from build123d import *

# Parameters (mm, degrees)
F1_DEPTH       = 18
F2_D           = 10
F3_D           = 10
F5_D           = 4
F5_CSINK_D     = 8.2
F5_CSINK_ANGLE = 90
F7_D           = 3
F7_DEPTH       = 20
F7_TIP         = 0.9012909285
F9_D           = 3
F9_DEPTH       = 20
F9_TIP         = 0.9012909285
F11_D          = 3
F11_DEPTH      = 20
F11_TIP        = 0.9012909285


with BuildPart() as f1:
    # F0 (on Right) → F1 (new body)
    with BuildSketch(Plane.YZ):
        Polygon((0, 230), (0, 0), (135, 0), (135, 206.1958576044), align=None)
    extrude(amount=F1_DEPTH)

    # F2 (through all)
    with Locations(Plane(origin=(0, 0, 0), x_dir=(0, 1, 0), z_dir=(-1, 0, 0))):
        with Locations((37.5, -170), (67.5, -170), (97.5, -170)):
            Hole(F2_D / 2)

    # F3 (through all)
    with Locations(Plane(origin=(0, 0, 0), x_dir=(0, 1, 0), z_dir=(-1, 0, 0))):
        with Locations((52.5, -190), (82.5, -190)):
            Hole(F3_D / 2)

    # F5 (through all)
    with Locations(Plane.YZ.offset(18)):
        with Locations((25, 27)):
            CounterSinkHole(F5_D / 2, F5_CSINK_D / 2, counter_sink_angle=F5_CSINK_ANGLE)

    # F7
    with Locations(Plane(origin=(0, 135, 0), x_dir=(-1, 0, 0), z_dir=(0, 1, 0))):
        with Locations((-9, 27), (-9, 106), (-9, 185)):
            Hole(F7_D / 2, depth=F7_DEPTH)
            with Locations((0, 0, -(F7_DEPTH + F7_TIP / 2))):  # 118° drill point
                Cone(0, F7_D / 2, F7_TIP, mode=Mode.SUBTRACT)

    # F9
    with Locations(Plane.XZ):
        with Locations((9, 197), (9, 112), (9, 27)):
            Hole(F9_D / 2, depth=F9_DEPTH)
            with Locations((0, 0, -(F9_DEPTH + F9_TIP / 2))):  # 118° drill point
                Cone(0, F9_D / 2, F9_TIP, mode=Mode.SUBTRACT)

    # F11
    with Locations(Plane(origin=(0, 39.3323164825, 223.0646513904), x_dir=(1, 0, 0), z_dir=(0, 0.1736481777, 0.984807753))):
        with Locations((9, -10.8564882588), (9, 79.1435117412)):
            Hole(F11_D / 2, depth=F11_DEPTH)
            with Locations((0, 0, -(F11_DEPTH + F11_TIP / 2))):  # 118° drill point
                Cone(0, F11_D / 2, F11_TIP, mode=Mode.SUBTRACT)


solid = f1.part
The model under review builds one solid part; all positions refer to its coordinate system, in mm. Coordinates: 2 decimals unless noted, no trailing zeros. Write each loop counter-clockwise with the first axis right and the second up, starting at its lowest first coordinate (ties: lowest second). Pieces come first, ordered by that corner, then holes. Notation, with made-up numbers: (62, -15) - (76, -15) arc R9 cw to (76, -10) - close; hole circle Ø8 at (-19, -28). An arc over 180 degrees is marked (long way). Answer as a JSON object with one key per item and string values. Group by question number.
1. Add section B-B (y = 37.5). Give the boundary of the cut face in (x, z).
2. Clearance check with flat-ended pins moving along their axes: pin 1 Ø2.5 at (y, z) = (25, 27) entering from -X; pin 2 Ø2.5 at (x, z) = (9, 27) entering from +Y; pin 3 Ø4 at (x, y) = (8.5, 41) entering from +Z; pin 4 Ø1.8 at (x, z) = (9, 112) entering from -Y. State where each tip first meets the part, or that it passes through.
3. Mouldability with a two-part tool opening along Z and no side actions: class faces 1 (the face through (9.126, 68.151, 165.043)), 2 (the face through (0, 67, 117)), 3 (the face through (9, 67, 0)) as pulls with the +Z half, pulls with the -Z half, needs draft (parallel to the pull), parting line crosses it, or undercut.
4. Add section A-A (z = 170). Give the boundary of the cut face in (x, y).
5. To check wall thickness, follow probe 1 along Y at (x, z) = (13.75, 190); probe 2 along Y at (x, z) = (5.25, 170); probe 3 along X at (y, z) = (14.75, 112). State the ranges of each line that lie inside material, in increasing order.
6. Add section C-C (y = 123.5). Give the boundary of the cut face in (x, z).
7. Add section D-D (y = 82). Give the boundary of the cut face in (x, z).
Findings:
{
 "1": {"outline": "(0, 0) - (18, 0) - (18, 165) - (0, 165) - close; (0, 175) - (18, 175) - (18, 223.39) - (0, 223.39) - close"},
 "2": {"pin 1": "through", "pin 2": "y = 114.85", "pin 3": "z = 223.12", "pin 4": "y = 20.36"},
 "3": {"face 1": "undercut", "face 2": "needs draft", "face 3": "pulls with the -Z half"},
 "4": {"outline": "(0, 0) - (18, 0) - (18, 32.5) - (0, 32.5) - close; (0, 42.5) - (18, 42.5) - (18, 62.5) - (0, 62.5) - close; (0, 72.5) - (18, 72.5) - (18, 92.5) - (0, 92.5) - close; (0, 102.5) - (18, 102.5) - (18, 135) - (0, 135) - close"},
 "5": {"probe 1": "0 to 47.5, 57.5 to 77.5, 87.5 to 135", "probe 2": "0 to 32.5, 42.5 to 62.5, 72.5 to 92.5, 102.5 to 135", "probe 3": "0 to 7.5, 10.5 to 18"},
 "6": {"outline": "(0, 0) - (18, 0) - (18, 208.22) - (0, 208.22) - close; hole circle Ø3 at (9, 27); hole circle Ø3 at (9, 106); hole circle Ø3 at (9, 185)"},
 "7": {"outline": "(0, 0) - (18, 0) - (18, 185.03) - (0, 185.03) - close; (0, 194.97) - (18, 194.97) - (18, 215.54) - (0, 215.54) - close"}
}
